Autodesk Inventor part; units mm, degrees
ref_plane "工作平面2" through (8, 0, 0) normal (1, 0, 0) x (0, 0, -1)
ref_plane "YZ Plane" through (0, 0, 0) normal (1, 0, 0) x (0, 1, 0)
ref_plane "XZ Plane" through (0, 0, 0) normal (0, 1, 0) x (-1, 0, 0)
sketch "草图1" plane through (0, 0, 0) normal (1, 0, 0) x (0, 1, 0)
  circle A0 centre (0, 0) radius 2
  circle A1 centre (0, 0) radius 5
  dimension "d0" = 4
  dimension "d1" = 10
extrude "拉伸1" add sketch "草图1" along normal blind 5 contours A0 | A1
extrude "拉伸2" add sketch "草图1" against normal blind 9 contours A0
chamfer "倒角1" distance 1 angle 45 1 edges at (-9, -2, 0)
thread "螺纹1"
ref_plane "工作平面2" through (8, 0, 0) normal (1, 0, 0) x (0, 0, -1)
ref_plane "工作平面1" through (6.5, 0, 0) normal (1, 0, 0) x (0, 0, -1)
sketch "草图3" plane through (8, 0, 0) normal (1, 0, 0) x (0, 0, -1)
  circle A0 centre (0, 0) radius 4
  dimension "d14" = 8
extrude "拉伸3" add sketch "草图3" along normal blind 2
chamfer "倒角3" distance 1 angle 45 1 edges at (5, -5, 0)
sketch "草图4" plane through (6.5, 0, 0) normal (1, 0, 0) x (0, 0, -1)
  circle A0 centre (0, 0) radius 2.5
  dimension "d29" = 5
loft "放样2" add profiles "草图4" section 1 edges at (5, -4, 0) section 3 edges at (8, 0, 4)
chamfer "倒角4" distance 0.5 angle 45 1 edges at (10, 0, 4)
sketch "草图6" plane through (10, 0, 0) normal (1, 0, 0) x (0, 0, -1)
  circle A0 centre (0, 0) radius 1.6
  line L0 (1.599, -0.9232) -> (0, -1.8464)
  line L1 (0, -1.8464) -> (-1.599, -0.9232)
  line L2 (-1.599, -0.9232) -> (-1.599, 0.9232)
  line L3 (-1.599, 0.9232) -> (0, 1.8464)
  line L4 (0, 1.8464) -> (1.599, 0.9232)
  line L5 (1.599, 0.9232) -> (1.599, -0.9232)
  dimension "d46" = 3.2
extrude "拉伸5" cut sketch "草图6" against normal blind 4
chamfer "倒角6" distance 0.2 angle 45 6 edges at (10, 1.3848, -0.7995) (10, 1.3848, 0.7995) (10, 0, 1.599) (10, -1.3848, 0.7995) (10, -1.3848, -0.7995) (10, 0, -1.599)
chamfer "倒角7" distance 0.2 angle 45 6 edges at (6, 1.3848, 0.7995) (6, 1.3848, -0.7995) (6, 0, 1.599) (6, -1.3848, 0.7995) (6, -1.3848, -0.7995) (6, 0, -1.599)
properties part number "knob" material "铝 6061-AHC"
Build history of the part. All positions in model axes, mm. A direction names the side the tool comes from. Round coordinates to 2 decimals unless told otherwise and drop trailing zeros. Loops run counter-clockwise (first coordinate to the right, second up) from the corner with the lowest first, then second, coordinate; pieces in that order, holes last.
Item 1: Drill centre lines: line 1 along X through (y, z) = (-1, -2.5); line 2 along X through (y, z) = (2.5, -0.75); line 3 along X through (y, z) = (0, 0.75). Where is each one in solid material? Low to high.
Item 2: Saw through at B-B (x = -4.25). List the corners of the cut face in (y, z), then the cut area to 3 significant figures.
Item 3: Saw through at C-C (x = 3.25). List the corners of the cut face in (y, z).
Item 4: Saw through at A-A (x = 9). List the corners of the cut face in (y, z), then the cut area to 3 significant figures.
Item 5: Which spindle directions (+Z, -Z, +X, -X, +Y, -Y) get a long thin tool onto all of the face, cutting with end or side? Do faces 1 (the face through (-4, 0, -2)), 2 (the face through (-9, 0, 0)), 3 (the face through (8.03, -1.39, 0.79)). Say none if no direction does.
Item 6: Pin check, flat tips, straight feed: P1, Ø0.9, axis at x = 8, y = 0, coming from the +Z side; P2, Ø2, axis at x = -6.5, z = -1, coming from the +Y side; P3, Ø1, axis at x = 2.5, y = 2, coming from the +Z side. Stop position of each tip, or through.
Worked answers:
1. line 1: x = 0 to 5.96, 7.04 to 10
1. line 2: x = 0 to 6.09, 6.91 to 10
1. line 3: x = -9 to 6
2. outline: circle Ø4 at (0, 0)
2. area: 12.6 mm2
3. outline: circle Ø10 at (0, 0)
4. outline: circle Ø8 at (0, 0); hole (-1.85, 0) - (-0.92, -1.6) - (0.92, -1.6) - (1.85, 0) - (0.92, 1.6) - (-0.92, 1.6) - close
4. area: 41.4 mm2
5. face 1: -X
5. face 2: +Z, -Z, -X, +Y, -Y
5. face 3: +X
6. P1: stops at z = 4
6. P2: stops at y = 2
6. P3: stops at z = 4.77
